Can you work these out from the model? Positions are in its coordinate system, mm. A direction names the side the tool comes from. Coordinates: 2 decimals unless noted, no trailing zeros. Order: outer loops, then holes, each group sorted by start corner. A loop starts at its lowest first (then second) coordinate and runs counter-clockwise, first axis right, second up. Notation, with made-up numbers: (58.25, 84) -> (88.25, 84) arc R30 cw to (88.25, 119) -> close; hole circle Ø4 at (-36, 39). An arc over 180 degrees is marked (long way). Return JSON: item names as keys, results as strings. Group by question number.
1) If we section it at B-B, the plane x = 35: Please give me the cut outline in (y, z).
2) Thinking about a two-plate mould opening in X: for faces 1 (the cylindrical face through (-56.69, 2.54, 0.99)), 2 (the flat face through (-52, 27, 2)), 3 (the cylindrical face through (1.099, -49.988, 0.986)), 4 (the cylindrical face through (1.385, 115.985, 0.986)), which applies, +X half, -X half, draft (parallel to the pull), parting line (faces both ways), or undercut?
3) For pin 1 (4 mm diameter, centred on x = 58, y = 47.5, fed in from -Z); pin 2 (1 mm diameter, centred on y = 85.5, z = 0.5, fed in from -X), each with a flat end and sliding along its axis, tell me the tip position at first contact or that it passes through.
4) If I drill on probe 1 along X at (y, z) = (43, 1.6); probe 2 along Y at (x, z) = (0, 0.9); probe 3 along X at (y, z) = (84.5, 1.45), over which ranges is the centre line in solid material (lowest first)? Write a range as from..to.
5) If we section it at D-D, the plane z = 0.8: State how many separate pieces and enclosed holes the cut face has, then the cut area to 3 significant figures.
6) If we section it at C-C, the plane y = -39.5: Please give me the cut outline in (x, z).
7) For faces 5 (the cylindrical face through (-1.385, -62.985, 0.986)), 6 (the cylindrical face through (-1.099, 102.988, 0.986)), which set-ups out of +Z, -Z, +X, -X, +Y, -Y let a thin tool reach every point of the face, with its end or its side?
8) If we section it at A-A, the plane y = 14: Please give me the cut outline in (x, z), then the cut area to 3 significant figures.
from build123d import *

# Parameters (mm, degrees)
F0_R     = 2.5
F1_DEPTH = 2


with BuildPart() as f1:
    # F0 (on Top) → F1 (new body)
    with BuildSketch(Plane.XY):
        with BuildLine():
            ThreePointArc((-50, 0), (0, -50), (50, 0))
            Line((50, 0), (50, 53))
            ThreePointArc((50, 53), (0, 103), (-50, 53))
            Line((-50, 53), (-50, 26.5))
            Line((-50, 26.5), (-50, 0))
        make_face()
        with BuildLine():
            Line((-63, 53), (-63, 26.5))
            Line((-63, 26.5), (-63, 0))
            ThreePointArc((-63, 0), (0, -63), (63, 0))
            Line((63, 0), (63, 53))
            ThreePointArc((63, 53), (0, 116), (-63, 53))
        make_face()
        with Locations((-44, -39.5)):
            Circle(F0_R, mode=Mode.SUBTRACT)
        with Locations((-59, 3.5)):
            Circle(F0_R, mode=Mode.SUBTRACT)
        with Locations((44, -39.5)):
            Circle(F0_R, mode=Mode.SUBTRACT)
        with Locations((58, 1.5)):
            Circle(F0_R, mode=Mode.SUBTRACT)
        with Locations((-58, 48.5)):
            Circle(F0_R, mode=Mode.SUBTRACT)
        with Locations((-42, 92.5)):
            Circle(F0_R, mode=Mode.SUBTRACT)
        with BuildLine():
            Line((50, 53), (50, 0))
            ThreePointArc((50, 0), (0, -50), (-50, 0))
            Line((-50, 0), (-50, 26.5))
            Line((-50, 26.5), (-50, 53))
            ThreePointArc((-50, 53), (0, 103), (50, 53))
        make_face(mode=Mode.SUBTRACT)
        with Locations((58, 47.5)):
            Circle(F0_R, mode=Mode.SUBTRACT)
        with Locations((43, 92.5)):
            Circle(F0_R, mode=Mode.SUBTRACT)
    extrude(amount=F1_DEPTH)


solid = f1.part
Result sheet:
{
 "1": {"outline": "(-52.38, 0) -> (-35.71, 0) -> (-35.71, 2) -> (-52.38, 2) -> close; (88.71, 0) -> (105.38, 0) -> (105.38, 2) -> (88.71, 2) -> close"},
 "2": {"face 1": "undercut", "face 2": "draft", "face 3": "undercut", "face 4": "parting line"},
 "3": {"pin 1": "passes through", "pin 2": "stops at x = -54.27"},
 "4": {"probe 1": "x = -63..-50, 50..63", "probe 2": "y = -63..-50, 103..116", "probe 3": "x = -54.56..-38.83, 38.83..54.56"},
 "5": {"separate pieces": "1", "enclosed holes": "9", "area": "5,840 mm2"},
 "6": {"outline": "(-49.08, 0) -> (-46.5, 0) -> (-46.5, 2) -> (-49.08, 2) -> close; (-41.5, 0) -> (-30.66, 0) -> (-30.66, 2) -> (-41.5, 2) -> close; (30.66, 0) -> (41.5, 0) -> (41.5, 2) -> (30.66, 2) -> close; (46.5, 0) -> (49.08, 0) -> (49.08, 2) -> (46.5, 2) -> close"},
 "7": {"face 5": "+Z, -Z, -Y", "face 6": "+Z, -Z"},
 "8": {"outline": "(-63, 0) -> (-50, 0) -> (-50, 2) -> (-63, 2) -> close; (50, 0) -> (63, 0) -> (63, 2) -> (50, 2) -> close", "area": "52.0 mm2"}
}
